Verification items for the finished model (mm, model axes). Face numbers are marked on the shaded views. A direction names the side the tool comes from. Round coordinates to 2 decimals unless told otherwise and drop trailing zeros. Write each loop counter-clockwise with the first axis right and the second up, starting at its lowest first coordinate (ties: lowest second). Pieces come first, ordered by that corner, then holes.
from build123d import *

# Parameters (mm, degrees)
F1_DEPTH = 8
F2_W     = 9.163002
F2_H     = 2
F3_DEPTH = 5
F4_R     = 0.6
F5_DEPTH = 6.001
F6_R     = 1
F7_DEPTH = 2
F8_R     = 0.85
F9_DEPTH = 3.001


with BuildPart() as f1:
    # F0 (on Top) → F1 (new body)
    with BuildSketch(Plane.XY):
        with BuildLine():
            Line((2.645751, 3), (-2.645751, 3))
            ThreePointArc((-2.645751, 3), (-4, 0), (-2.645751, -3))
            Line((-2.645751, -3), (2.645751, -3))
            ThreePointArc((2.645751, -3), (4, 0), (2.645751, 3))
        make_face()
    extrude(amount=F1_DEPTH)

    # F2 (on face) → F3 (cut)
    with BuildSketch(Plane.XY.offset(8)):
        Rectangle(F2_W, F2_H)
    extrude(amount=-F3_DEPTH, mode=Mode.SUBTRACT)

    # F4 (on face) → F5 (cut, through all)
    with BuildSketch(Plane.XZ.offset(3)):
        with Locations((0, 5.5)):
            Circle(F4_R)
    extrude(amount=-F5_DEPTH, mode=Mode.SUBTRACT)

    # F6 (on face) → F7 (cut, through all)
    with BuildSketch(Plane(origin=(0, 3, 0), x_dir=(-1, 0, 0), z_dir=(0, 1, 0))):
        with Locations((0, 5.5)):
            Circle(F6_R)
    extrude(amount=-F7_DEPTH, mode=Mode.SUBTRACT)

    # F8 (on face) → F9 (cut, through all)
    with BuildSketch(Plane.XY.offset(3)):
        Circle(F8_R)
    extrude(amount=-F9_DEPTH, mode=Mode.SUBTRACT)


solid = f1.part
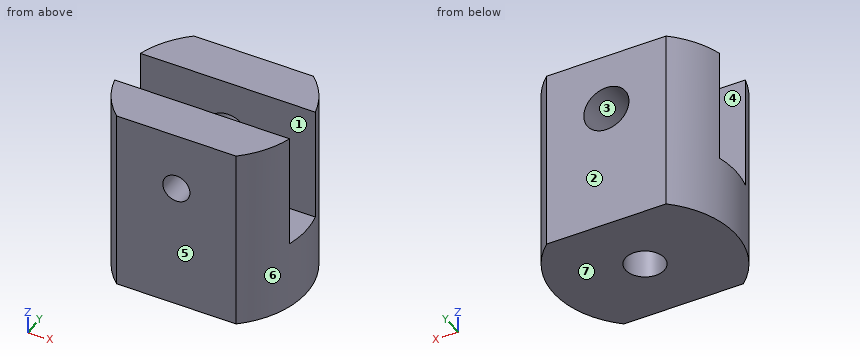
Q1. Sectioned sample at D-D (z = 3.25). Enter the section's corners in (x, y).
Recorded:
outline: (-3.87, -1) arc R4 ccw to (-2.65, -3) - (2.65, -3) arc R4 ccw to (3.87, -1) - close; (-3.87, 1) - (3.87, 1) arc R4 ccw to (2.65, 3) - (-2.65, 3) arc R4 ccw to start
Q2. Tool access check on the marked faces 1, 2 and 3. Record the directions out of +Z, -Z, +X, -X, +Y, -Y that give a thin tool (end or side, any length) a straight path to the whole face; none if there is none.
Recorded:
face 1: +Z, +X, -X
face 2: +Z, -Z, +X, -X, +Y
face 3: +Y
Q3. Release check for a two-part mould opening along Y. For the marked faces 4, 5, 6 and 7 record: released by +Y, released by -Y, zero draft, split by the parting line, or undercut.
Recorded:
face 4: undercut
face 5: released by -Y
face 6: split by the parting line
face 7: zero draft
Q4. Sectioned sample at C-C (z = 5.5). Enter the section's corners in (x, y), plus the area to 3 significant figures.
Recorded:
outline: (-3.87, -1) arc R4 ccw to (-2.65, -3) - (-0.6, -3) - (-0.6, -1) - close; (-3.87, 1) - (-1, 1) - (-1, 3) - (-2.65, 3) arc R4 ccw to start; (0.6, -3) - (2.65, -3) arc R4 ccw to (3.87, -1) - (0.6, -1) - close; (1, 1) - (3.87, 1) arc R4 ccw to (2.65, 3) - (1, 3) - close
area: 20.8 mm2
Q5. Sectioned sample at B-B (x = 0). Enter the section's corners in (y, z), plus the area to 3 significant figures.
Recorded:
outline: (-3, 0) - (-0.85, 0) - (-0.85, 3) - (-1, 3) - (-1, 4.9) - (-3, 4.9) - close; (-3, 6.1) - (-1, 6.1) - (-1, 8) - (-3, 8) - close; (0.85, 0) - (3, 0) - (3, 4.5) - (1, 4.5) - (1, 3) - (0.85, 3) - close; (1, 6.5) - (3, 6.5) - (3, 8) - (1, 8) - close
area: 26.5 mm2
Q6. Sectioned sample at A-A (y = 0). Enter the section's corners in (x, z).
Recorded:
outline: (-4, 0) - (-0.85, 0) - (-0.85, 3) - (-4, 3) - close; (0.85, 0) - (4, 0) - (4, 3) - (0.85, 3) - close
Q7. Depth check by flat-ended pin: P1, Ø1, axis at x = 2, y = 0, coming from the +Z side; P2, Ø1.5, axis at y = 1, z = 6.5, coming from the +X side; P3, Ø1.8, axis at x = 0, z = 5.5, coming from the +Y side. Enter the tip coordinate at first touch or a pass-through.
Recorded:
P1: stops at z = 3
P2: stops at x = 3.87
P3: stops at y = -1
Q8. Material ranges on line 1 along Y through (x, z) = (0.25, 4.5); line 2 along Y through (x, z) = (3, 6.5); line 3 along Z through (x, y) = (-0.25, 1.5), recorded low to high.
Recorded:
line 1: y = -3 to -1, 1 to 3
line 2: y = -2.65 to -1, 1 to 2.65
line 3: z = 0 to 4.53, 6.47 to 8
